Check sheet for the modelled part. Datum: model origin and axes. Units: mm. A direction names the side the tool comes from. Round coordinates to 2 decimals unless told otherwise and drop trailing zeros. Loops run counter-clockwise (first coordinate to the right, second up) from the corner with the lowest first, then second, coordinate; pieces in that order, holes last. Notation, with made-up numbers: (25, 44) -> (73, 44) arc R23 ccw to (73, 61) -> close; hole circle Ø4 at (84, -10.5). An arc over 180 degrees is marked (long way). Use one line per item in the form item = value. Start each with the question number.
(1) Sectioned sample at C-C (x = 1212). Record the cut outline in (y, z) (3 decimals).
(2) Sectioned sample at A-A (z = -28.5). Record the cut outline in (x, y) (3 decimals).
(3) Sectioned sample at B-B (y = 32.5). Record the cut outline in (x, z) (3 decimals), and give its area (3 significant figures).
(4) Material ranges on probe 1 along Y at (x, z) = (218, -14.5) (3 decimals); probe 2 along Y at (x, z) = (88.9, -1.8); probe 3 along Z at (x, y) = (979, 14.5) (3 decimals), recorded low to high. Write a range as [from, to].
(5) Draft check along Y on faces 3 (the flat face through (801, 41.275, -22)), 4 (the flat face through (801, 3.175, -22)), 5 (the flat face through (801, 44.45, -22)), 6 (the flat face through (1625.6, 23, -42)). Enter one of: released by +Y, released by -Y, zero draft, split by the parting line, or undercut.
(6) Set-up check for faces 1 (the flat face through (801, 22, 0)), 2 (the flat face through (801, 22, -41.275)): record each of +Z, -Z, +X, -X, +Y, -Y from which the full face is reachable in a straight line by a thin tool's end or side.
from build123d import *

# Parameters (mm, degrees)
SKETCH1_W           = 44.45
SKETCH1_H           = 44.45
SKETCH1_W_2         = 38.1
SKETCH1_H_2         = 38.1
BOSS_EXTRUDE1_DEPTH = 1625.6
SKETCH2_R           = 3.3734375
CUT_EXTRUDE1_DEPTH  = 45.45


with BuildPart() as part:
    # Sketch1 → Boss-Extrude1 (new body)
    with BuildSketch(Plane(origin=(0, 0, 0), x_dir=(0, 0, -1), z_dir=(1, 0, 0))):
        with Locations((22.225, 22.225)):
            Rectangle(SKETCH1_W, SKETCH1_H)
        with Locations((22.225, 22.225)):
            Rectangle(SKETCH1_W_2, SKETCH1_H_2, mode=Mode.SUBTRACT)
    extrude(amount=BOSS_EXTRUDE1_DEPTH)

    # Sketch2 → Cut-Extrude1 (cut, through all)
    with BuildSketch(Plane.XY):
        with Locations((784.225, 22.225)):
            Circle(SKETCH2_R)
        with Locations((815.975, 22.225)):
            Circle(SKETCH2_R)
        with Locations((571.5, 22.225)):
            Circle(SKETCH2_R)
        with Locations((88.9, 22.225)):
            Circle(SKETCH2_R)
    extrude(amount=-CUT_EXTRUDE1_DEPTH, mode=Mode.SUBTRACT)


solid = part.part
Checks:
q1.outline = (0, -44.45) -> (44.45, -44.45) -> (44.45, 0) -> (0, 0) -> close; hole (3.175, -41.275) -> (41.275, -41.275) -> (41.275, -3.175) -> (3.175, -3.175) -> close
q2.outline = (0, 0) -> (1625.6, 0) -> (1625.6, 3.175) -> (0, 3.175) -> close; (0, 41.275) -> (1625.6, 41.275) -> (1625.6, 44.45) -> (0, 44.45) -> close
q3.outline = (0, -44.45) -> (1625.6, -44.45) -> (1625.6, -41.275) -> (0, -41.275) -> close; (0, -3.175) -> (1625.6, -3.175) -> (1625.6, 0) -> (0, 0) -> close
q3.area = 10,300 mm2
q4.probe_1 = [0, 3.175], [41.275, 44.45]
q4.probe_2 = [0, 18.85], [25.6, 44.45]
q4.probe_3 = [-44.45, -41.275], [-3.175, 0]
q5.face_3 = undercut
q5.face_4 = undercut
q5.face_5 = released by +Y
q5.face_6 = zero draft
q6.face_1 = +Z, +X, -X, +Y, -Y
q6.face_2 = +X, -X
